Part print with two shaded views. Sizes in mm from the minimum x, y, z corner. Give positions to 0.01 mm unless a question says otherwise; leave off trailing zeros. Write each loop counter-clockwise with the first axis right and the second up, starting at its lowest first coordinate (ties: lowest second). Pieces come first, ordered by that corner, then holes. Notation, with made-up numbers: (85.25, 75.25) -> (89.25, 75.25) arc R16 cw to (89.25, 87.25) -> close; hole circle Ø6 at (2.25, -13). An arc over 180 degrees is marked (long way). Answer as a JSON object with one key per item and string values.
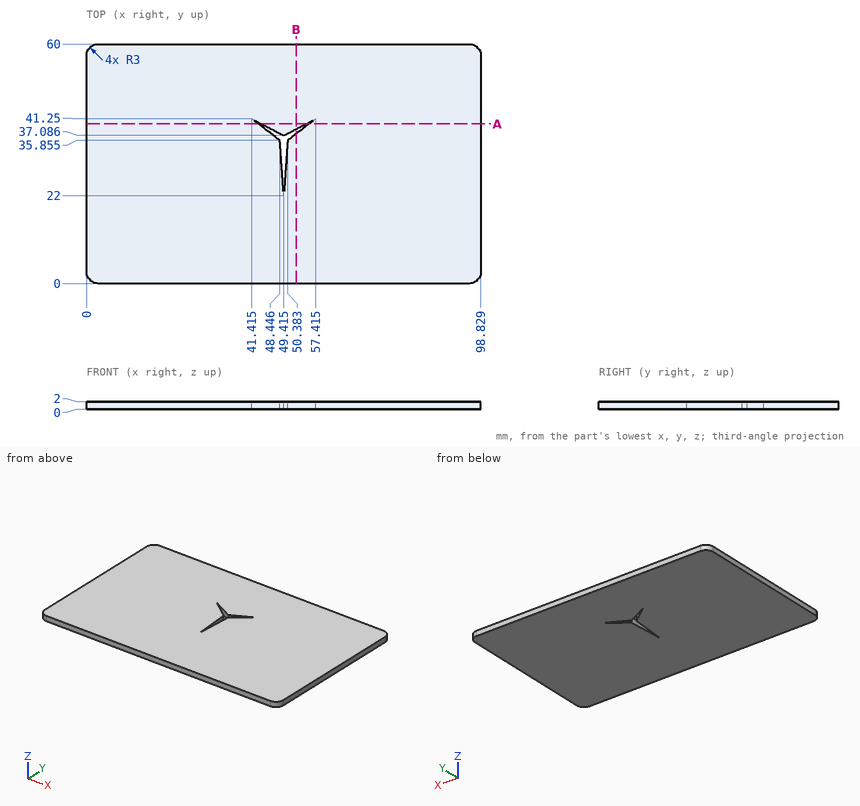
1) Slice it at B-B (x = 52.5). List the corners of the cut face in (y, z).
Model answer:
{"outline": "(0, 0) -> (37.48, 0) -> (37.48, 2) -> (0, 2) -> close; (38.69, 0) -> (60, 0) -> (60, 2) -> (38.69, 2) -> close"}
2) Slice it at A-A (y = 40). List the corners of the cut face in (x, z) (1 decimal).
Model answer:
{"outline": "(0, 0) -> (43, 0) -> (43, 2) -> (0, 2) -> close; (43.8, 0) -> (55, 0) -> (55, 2) -> (43.8, 2) -> close; (55.8, 0) -> (98.8, 0) -> (98.8, 2) -> (55.8, 2) -> close"}
3) Wall check: probe 1 along X at (y, z) = (25, 0.35) (1 decimal); probe 2 along X at (y, z) = (29, 0.8) (1 decimal); probe 3 along Y at (x, z) = (55, 1) (1 decimal). Give the ranges that are in metal, low to high.
Model answer:
{"probe 1": "x = 0 to 49.2, 49.6 to 98.8", "probe 2": "x = 0 to 48.9, 49.9 to 98.8", "probe 3": "y = 0 to 39.4, 40 to 60"}
